from build123d import *

# Parameters (mm, degrees)
F0_W     = 12
F0_H     = 12
F1_DEPTH = 4
F2_D     = 6
F2_DEPTH = 4.001
F3_D     = 6


with BuildPart() as f1:
    # F0 (on Top) → F1 (new body, symmetric)
    with BuildSketch(Plane.XY):
        with BuildLine():
            Line((459, -20), (459, 20))
            Line((459, 20), (-459, 20))
            Line((-459, 20), (-459, -5))
            ThreePointArc((-459, -5), (-454.6066017178, -15.6066017178), (-444, -20))
            Line((-444, -20), (459, -20))
        make_face()
        with Locations((-400, 0)):
            Rectangle(F0_W, F0_H, mode=Mode.SUBTRACT)
        with Locations((-300, 0)):
            Rectangle(F0_W, F0_H, mode=Mode.SUBTRACT)
        with Locations((-200, 0)):
            Rectangle(F0_W, F0_H, mode=Mode.SUBTRACT)
        with Locations((-100, 0)):
            Rectangle(F0_W, F0_H, mode=Mode.SUBTRACT)
        Rectangle(F0_W, F0_H, mode=Mode.SUBTRACT)
        with Locations((100, 0)):
            Rectangle(F0_W, F0_H, mode=Mode.SUBTRACT)
        with Locations((200, 0)):
            Rectangle(F0_W, F0_H, mode=Mode.SUBTRACT)
        with Locations((300, 0)):
            Rectangle(F0_W, F0_H, mode=Mode.SUBTRACT)
        with Locations((400, 0)):
            Rectangle(F0_W, F0_H, mode=Mode.SUBTRACT)
    extrude(amount=F1_DEPTH, both=True)

    # F2 (through all, one way)
    with BuildSketch(Plane.XY):
        with Locations((-444, -5)):
            Circle(F2_D / 2)
    extrude(amount=-F2_DEPTH, mode=Mode.SUBTRACT)

    # F3 (through all)
    with Locations(Plane(origin=(0, 0, 0), x_dir=(1, 0, 0), z_dir=(0, 0, -1))):
        with Locations((-444, 5)):
            Hole(F3_D / 2)


solid = f1.part
Verification items for the finished model (mm, model axes). Coordinates: 2 decimals unless noted, no trailing zeros. One line per item, written item: value. Start each with the question number.
Item 1: Gauge pin test, flat end, axial feed: pin 1 (1 mm diameter, centred on y = -12.5, z = 1.5, fed in from -X). Record the tip position at first contact, or that the pin passes through.
Item 2: Scan lines: probe 1 along Y at (x, z) = (-444, 1.2); probe 2 along Y at (x, z) = (304, 0); probe 3 along X at (y, z) = (-7.5, -1). Record each from-to range of solid material in increasing order.
Item 3: Sectioned sample at A-A (z = 1.5). Count the separate pieces of the cut face and the enclosed holes in it, then the cut area to 3 significant figures.
Conclusion:
1. pin 1: stops at x = -457.27
2. probe 1: y = -20 to -8, -2 to 20
2. probe 2: y = -20 to -6, 6 to 20
2. probe 3: x = -458.79 to -445.66, -442.34 to 459
3. separate pieces: 1
3. enclosed holes: 10
3. area: 35,300 mm^2
